from build123d import *

# Parameters (mm, degrees)
F0_R     = 35
F0_W     = 0.9
F0_H     = 8
F1_DEPTH = 80
F2_DEPTH = 78.8
F3_DEPTH = 37
F5_D     = 6
F6_DEPTH = 2.2
F7_DEPTH = 11.5
F8_R     = 2.5


with BuildPart() as f1:
    # F0 (on Top) → F1 (new body)
    with BuildSketch(Plane.XY):
        with BuildLine():
            ThreePointArc((5.8807484886, -19.4080062609), (45.7302931295, -34.0256498123), (71.105810187, 0))
            ThreePointArc((71.105810187, 0), (45.7302931295, 34.0256498123), (5.8807484886, 19.4080062609))
            ThreePointArc((5.8807484886, 19.4080062609), (1.580160384, 10.1244829736), (0.105810187, 6.5e-08))
            ThreePointArc((0.105810187, 6.5e-08), (1.5801603655, -10.1244829114), (5.8807484886, -19.4080062609))
        make_face()
        with Locations((35.605810187, 0)):
            Circle(F0_R, mode=Mode.SUBTRACT)
        with BuildLine():
            Line((-1.8941865764, -7.5000121373), (5.8807484886, -19.4080062609))
            ThreePointArc((5.8807484886, -19.4080062609), (1.5801603655, -10.1244829114), (0.105810187, 6.5e-08))
            Line((0.105810187, 6.5e-08), (0.105810187, -7.4964140307))
            Line((0.105810187, -7.4964140307), (-1.8941865764, -7.5000121373))
        make_face()
        with BuildLine():
            ThreePointArc((0.105810187, 6.5e-08), (1.580160384, 10.1244829736), (5.8807484886, 19.4080062609))
            Line((5.8807484886, 19.4080062609), (-1.8941865764, 7.5000121373))
            Line((-1.8941865764, 7.5000121373), (-0.9941865764, 7.5016312878))
            Line((-0.9941865764, 7.5016312878), (0.105810187, 7.5016312878))
            Line((0.105810187, 7.5016312878), (0.105810187, 6.5e-08))
        make_face()
        with Locations((35.605810187, 0)):
            Circle(F0_R)
        Polygon((-0.9941865764, 7.5016312878), (-1.8941865764, 7.5000121373), (-1.8941865764, 4.0026086286), (-0.9941865764, 4.0026086286), align=None)
        Polygon((-1.8941865764, -3.9973913714), (-1.8941865764, -7.5000121373), (0.105810187, -7.4964140307), (-0.9941865764, -7.4964140307), (-0.9941865764, -3.9973913714), align=None)
        Polygon((0.105810187, -7.4964140307), (0.105810187, 6.5e-08), (0.105810187, 7.5016312878), (-0.9941865764, 7.5016312878), (-0.9941865764, 4.0026086286), (-0.0941865764, 4.0026086286), (-0.0941865764, -3.9973913714), (-0.9941865764, -3.9973913714), (-0.9941865764, -7.4964140307), align=None)
        with Locations((-0.5441865764, 0.0026086286)):
            Rectangle(F0_W, F0_H)
        with Locations((-1.4441865764, 0.0026086286)):
            Rectangle(F0_W, F0_H)
    extrude(amount=F1_DEPTH)

    # F0 (on Top) → F2 (cut)
    with BuildSketch(Plane.XY):
        with Locations((35.605810187, 0)):
            Circle(F0_R)
    extrude(amount=F2_DEPTH, mode=Mode.SUBTRACT)

    # F0 (on Top) → F3 (cut)
    with BuildSketch(Plane.XY):
        with Locations((-0.5441865764, 0.0026086286)):
            Rectangle(F0_W, F0_H)
        Polygon((0.105810187, -7.4964140307), (0.105810187, 6.5e-08), (0.105810187, 7.5016312878), (-0.9941865764, 7.5016312878), (-0.9941865764, 4.0026086286), (-0.0941865764, 4.0026086286), (-0.0941865764, -3.9973913714), (-0.9941865764, -3.9973913714), (-0.9941865764, -7.4964140307), align=None)
        with Locations((-1.4441865764, 0.0026086286)):
            Rectangle(F0_W, F0_H)
    extrude(amount=F3_DEPTH, mode=Mode.SUBTRACT)

    # F5 (through all)
    with Locations(Plane.XY.offset(80)):
        with Locations((35.605810187, 0)):
            Hole(F5_D / 2)

    # F0 (on Top) → F6 (cut)
    with BuildSketch(Plane.XY):
        Polygon((-1.8941865764, -3.9973913714), (-1.8941865764, -7.5000121373), (0.105810187, -7.4964140307), (-0.9941865764, -7.4964140307), (-0.9941865764, -3.9973913714), align=None)
        Polygon((-0.9941865764, 7.5016312878), (-1.8941865764, 7.5000121373), (-1.8941865764, 4.0026086286), (-0.9941865764, 4.0026086286), align=None)
    extrude(amount=F6_DEPTH, mode=Mode.SUBTRACT)

    # F7 (add): a face of the model
    f7_faces = [f1.faces().sort_by_distance(p)[0] for p in [
        (-0.7480133578, 0.0026086286, 37),
    ]]
    extrude(f7_faces, amount=F7_DEPTH)

    # F8
    f8_edges = [f1.edges().sort_by_distance(p)[0] for p in [
        (0.60581, 0, 78.8),
    ]]
    fillet(f8_edges, radius=F8_R)


solid = f1.part
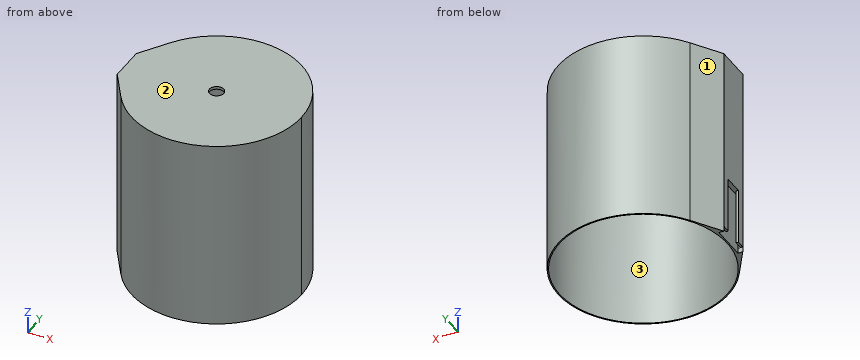
Input: part model. Units: mm. Frame: model coordinates. Face numbers are marked on the shaded views. Give positions to 0.01 mm unless a question says otherwise; leave off trailing zeros. Write each loop counter-clockwise with the first axis right and the second up, starting at its lowest first coordinate (ties: lowest second). Pieces come first, ordered by that corner, then holes. Notation, with made-up numbers: (24, 67) -> (80, 67) arc R35 cw to (80, 100) -> close; hole circle Ø5 at (89.25, 40). An arc over 180 degrees is marked (long way). Use one line per item in the form item = value. Start each with the question number.
1) Section query A-A on z = 19. Return the cut outline in (x, y).
2) Draft query along X for the marked faces 1, 2 and 3. Return one class per face: pulls with the +X half, pulls with the -X half, needs draft (parallel to the pull), parting line crosses it, or undercut.
3) Section query B-B on z = 28.5. Return the cut outline in (x, y), then the cut area to 3 significant figures.
4) Ray query, probe 1 along Y at (x, z) = (35.5, 69); probe 2 along Z at (x, y) = (61, -11.5); probe 3 along Y at (x, z) = (30, 23.5). Return the intervals inside material, ascending. Write a range as from..to.
5) Pin query (flat end, axial travel): pin 1 (1 mm diameter, centred on x = -1.5, z = 11.5, fed in from +Y); pin 2 (1.2 mm diameter, centred on x = -0.5, z = 19, fed in from -Y); pin 3 (3 mm diameter, centred on y = -18, z = 43, fed in from -X). Return the tip coordinate at first contact, or that it passes through.
Outcome:
q1.outline = (-1.89, -7.5) -> (5.88, -19.41) arc R35.5 ccw (long way) to (5.88, 19.41) -> (-1.89, 7.5) -> (-1.89, 4) -> (-0.99, 4) -> (-0.99, 7.5) -> (0.11, 7.5) -> (0.11, -7.5) -> (-0.99, -7.5) -> (-0.99, -4) -> (-1.89, -4) -> close; hole circle Ø70 at (35.61, 0)
q2.face_1 = pulls with the -X half
q2.face_2 = needs draft
q2.face_3 = undercut
q3.outline = (-1.89, -7.5) -> (5.88, -19.41) arc R35.5 ccw (long way) to (5.88, 19.41) -> (-1.89, 7.5) -> close; hole circle Ø70 at (35.61, 0)
q3.area = 168 mm^2
q4.probe_1 = -35.5..-35, 35..35.5
q4.probe_2 = 78.8..80
q4.probe_3 = -35.05..-34.55, 34.55..35.05
q5.pin_1 = 8.87
q5.pin_2 = -10.55
q5.pin_3 = 3.98
